Geometry check sheet. Reference: the model listing, model coordinates, mm. Face numbers are marked on the shaded views. A direction names the side the tool comes from. Coordinates: 2 decimals unless noted, no trailing zeros. Order: outer loops, then holes, each group sorted by start corner. A loop starts at its lowest first (then second) coordinate and runs counter-clockwise, first axis right, second up. Notation, with made-up numbers: (10.25, 15) - (14.25, 15) arc R34 cw to (14.25, 45) - close; hole circle Ø4 at (69.5, 78). An arc over 180 degrees is marked (long way). Return JSON: item names as keys, results as strings. Group by question number.
Item 1: Gauge pin test, flat ends, axial feed: pin 1 (1.8 mm diameter, centred on y = 0, z = -5.16, fed in from +X); pin 2 (12 mm diameter, centred on x = 37.5, y = -0.5, fed in from +Z); pin 3 (1 mm diameter, centred on x = 19, y = -8, fed in from -Z); pin 4 (3 mm diameter, centred on x = 33, y = -4, fed in from +Z). Record the tip position at first contact, or that the pin passes through.
Item 2: Draft check along X on the marked faces 4, 5 and 6. Enter one of: pulls with the +X half, pulls with the -X half, needs draft (parallel to the pull), parting line crosses it, or undercut.
Item 3: Scan lines: probe 1 along Z at (x, y) = (4.75, 0); probe 2 along X at (y, z) = (6, -0.75); probe 3 along Z at (x, y) = (43.5, 0.25). Record each from-to range of solid material in increasing order.
Item 4: Section check B-B on x = -7. Enter the section's corners in (y, z).
Item 5: Tool access check on the marked faces 1, 2 and 3. Record the directions out of +Z, -Z, +X, -X, +Y, -Y that give a thin tool (end or side, any length) a straight path to the whole face; none if there is none.
Item 6: Section check A-A on x = 30. Enter the section's corners in (y, z), then the cut area to 3 significant figures.
from build123d import *

# Parameters (mm, degrees)
TROU_TARAUD_M2X0_41_D           = 1.6
TROU_TARAUD_M2X0_41_DEPTH       = 6
TROU_TARAUD_M2X0_41_CSINK_D     = 2.05
TROU_TARAUD_M2X0_41_CSINK_ANGLE = 90
TROU_TARAUD_M2X0_41_TIP         = 0.480688495


with BuildPart() as part:
    # Esquisse1 → Révolution1 (revolve)
    with BuildSketch(Plane.XY):
        Polygon((-14, 1.15), (0, 1.15), (0, 9), (9, 9), (9, 6), (18, 6), (18, 9), (22, 13), (45, 13), (45, 3.5), (47, 3.5), (47, 0), (-14, 0), align=None)
    revolve(axis=Axis((-25.880121982, 0, 0), (1, 0, 0)))

    # Trou taraudé M2x0.41
    with Locations(Plane.ZY):
        with Locations((0, 5.164935058), (5.164935058, 0), (0, -5.164935058), (-5.164935058, 0)):
            CounterSinkHole(TROU_TARAUD_M2X0_41_D / 2, TROU_TARAUD_M2X0_41_CSINK_D / 2, depth=TROU_TARAUD_M2X0_41_DEPTH, counter_sink_angle=TROU_TARAUD_M2X0_41_CSINK_ANGLE)
            with Locations((0, 0, -(TROU_TARAUD_M2X0_41_DEPTH + TROU_TARAUD_M2X0_41_TIP / 2))):  # 118° drill point
                Cone(0, TROU_TARAUD_M2X0_41_D / 2, TROU_TARAUD_M2X0_41_TIP, mode=Mode.SUBTRACT)


solid = part.part
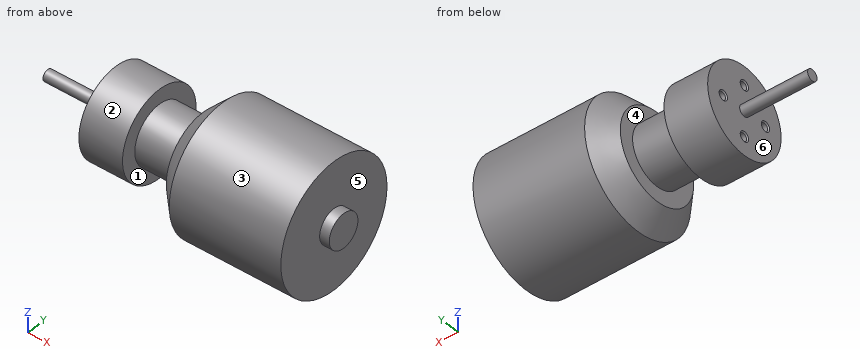
Computed:
{
 "1": {"pin 1": "stops at x = 45", "pin 2": "stops at z = 13", "pin 3": "stops at z = -6.99", "pin 4": "stops at z = 12.76"},
 "2": {"face 4": "undercut", "face 5": "pulls with the +X half", "face 6": "pulls with the -X half"},
 "3": {"probe 1": "z = -9 to -5.96, -4.36 to 4.36, 5.96 to 9", "probe 2": "x = 0 to 9, 18 to 45", "probe 3": "z = -13 to 13"},
 "4": {"outline": "circle Ø2.3 at (0, 0)"},
 "5": {"face 1": "none", "face 2": "-X", "face 3": "+X, -X"},
 "6": {"outline": "circle Ø26 at (0, 0)", "area": "531 mm²"}
}
